Source: CAD feature listing. Evaluate the final solid. Frame: model axes, mm. Face numbers are marked on the shaded views. A direction names the side the tool comes from. Round coordinates to 2 decimals unless told otherwise and drop trailing zeros. Order: outer loops, then holes, each group sorted by start corner. A loop starts at its lowest first (then second) coordinate and runs counter-clockwise, first axis right, second up. Notation, with made-up numbers: (-22, 57.25) - (-7, 57.25) arc R15 ccw to (-7, 77.25) - close; hole circle Ø10 at (26, 28.5). An arc over 180 degrees is marked (long way). Return JSON: item names as keys, results as strings. Group by question number.
1) Section C-C, the plane y = 7.5. Give the number of separate pieces and of enclosed holes in the cut face, plus the area to 3 significant figures.
2) Ray query, line 1 (X direction, y = 0, z = 4.1); line 2 (Y direction, x = 12.85, z = 0); line 3 (Y direction, x = 4.25, z = -1.5). Return the intervals inside material, ascending. Write a range as from..to.
3) Contact query for flat-ended pins moving along their axis: P1, Ø6, axis at x = 4.5, y = -3, coming from the +Z side; P2, Ø4, axis at y = 0, z = 0, coming from the +X side; P3, Ø3, axis at x = 4, z = -7, coming from the -Y side; P4, Ø5, axis at x = 7.5, y = 5, coming from the -Z side. Output: stop coordinate, or through.
4) Section B-B, the plane z = 0. Return loops of the section in (x, y).
5) Section A-A, the plane y = 0. Return loops of the section in (x, z), plus the area to 3 significant figures.
6) Mould query, pull axis Z, two halves, no side actions, for the marked faces 1, 2 and 3. Classes: pulls with the +Z half, pulls with the -Z half, needs draft (parallel to the pull), parting line crosses it, or undercut.
7) Access query for the marked faces 4, 5 and 6. Directions: +Z, -Z, +X, -X, +Y, -Y. A direction counts if a zero-diameter tool reaches every point of the face in a straight line with its end or side. Return the directions, or none.
Autodesk Inventor part; units mm, degrees
ref_plane "Work Plane1" through (20, 0, 0) normal (0, 0, -1) x (-1, 0, 0)
ref_plane "YZ Plane" through (0, 0, 0) normal (1, 0, 0) x (0, 1, 0)
ref_plane "XZ Plane" through (0, 0, 0) normal (0, 1, 0) x (-1, 0, 0)
sketch "Sketch1" plane through (0, 0, 0) normal (0, 0, 1) x (1, 0, 0)
  line L0 (0, 0) -> (20, 0)
  line L1 (0, 0) -> (0, 5)
  line L2 (0, 5) -> (0, 9)
  line L3 (0, 9) -> (2, 9)
  line L4 (20, 0) -> (20, 5)
  line L5 (20, 5) -> (0, 5)
  line L6 (15, 0) -> (15, 9)
  line L7 (15, 9) -> (13, 9)
  line L8 (13, 9) -> (10, 5)
  line L9 (2, 9) -> (13, 9) construction
  line L10 (7.5, 9) -> (7.5, -5.2368) construction
  line L11 (2, 9) -> (5, 5)
  point P0 (17.5, 0)
  point P1 (15, 5)
  dimension "d0" = 20
  dimension "d2" = 5
  dimension "d3" = 4
  dimension "d4" = 2
  dimension "d9" = 9
  dimension "d10" = 5
  dimension "d11" = 2
  dimension "d12" = 2.5
  dimension "d13" = 20
revolve "Revolution1" add sketch "Sketch1" angle 360 about axis through (0, 0, 0) along (1, 0, 0)
sketch "Sketch2" plane through (0, 0, 0) normal (-1, 0, 0) x (0, 0, 1)
  circle A0 centre (0, 0) radius 2.4
  circle A1 centre (0, 7.5) radius 0.5
  dimension "d15" = 4.8
  dimension "d21" = 1
  dimension "d22" = 7.5
extrude "Extrusion1" cut sketch "Sketch2" against normal blind 20
ref_plane "Work Plane1" through (20, 0, 0) normal (0, 0, -1) x (-1, 0, 0)
sketch "Sketch3" plane through (20, 0, 0) normal (0, 0, -1) x (-1, 0, 0)
  circle A0 centre (2.4908, 0) radius 1
  point P0 (20, 0)
  dimension "d18" = 2
extrude "Extrusion2" cut sketch "Sketch3" against normal blind 6
properties part number "stepper_spool"
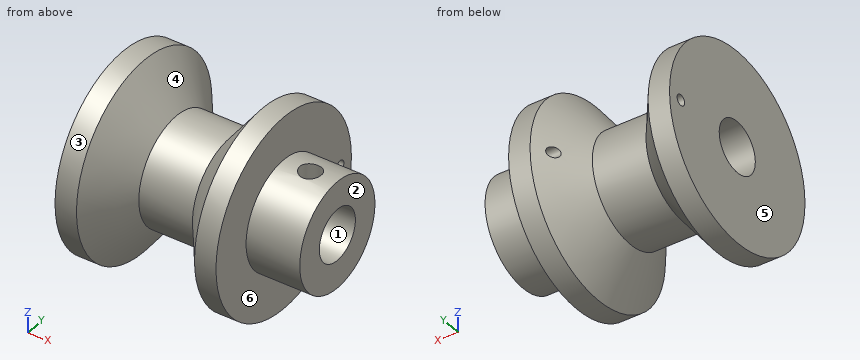
Geometry check:
{
 "1": {"separate pieces": "4", "enclosed holes": "0", "area": "48.2 mm2"},
 "2": {"line 1": "0..16.51, 18.51..20", "line 2": "-8.8..-2.4, 2.4..7, 8..8.8", "line 3": "-5.81..-1.87, 1.87..5.81"},
 "3": {"P1": "z = 8.9", "P2": "through", "P3": "y = -5.1", "P4": "z = -4.33"},
 "4": {"outline": "(0, -9) - (2, -9) - (5, -5) - (10, -5) - (13, -9) - (15, -9) - (15, -5) - (20, -5) - (20, -2.4) - (0, -2.4) - close; (0, 2.4) - (20, 2.4) - (20, 5) - (15, 5) - (15, 7) - (11.5, 7) - (10, 5) - (5, 5) - (3.5, 7) - (0, 7) - close; (0, 8) - (2.75, 8) - (2, 9) - (0, 9) - close; (12.25, 8) - (15, 8) - (15, 9) - (13, 9) - close"},
 "5": {"outline": "(0, -9) - (2, -9) - (5, -5) - (10, -5) - (13, -9) - (15, -9) - (15, -5) - (20, -5) - (20, -2.4) - (0, -2.4) - close; (0, 2.4) - (16.51, 2.4) - (16.51, 5) - (15, 5) - (15, 9) - (13, 9) - (10, 5) - (5, 5) - (2, 9) - (0, 9) - close; (18.51, 2.4) - (20, 2.4) - (20, 5) - (18.51, 5) - close", "area": "155 mm2"},
 "6": {"face 1": "undercut", "face 2": "needs draft", "face 3": "parting line crosses it"},
 "7": {"face 4": "none", "face 5": "+Z, -Z, -X, +Y, -Y", "face 6": "+X"}
}
